Job drawing, mm, ordinate dimensions from the low corner. One solid piece. Coordinates: 2 decimals unless noted, no trailing zeros. Write each loop counter-clockwise with the first axis right and the second up, starting at its lowest first coordinate (ties: lowest second). Pieces come first, ordered by that corner, then holes. Notation, with made-up numbers: (53, 21) - (106, 21) arc R15 cw to (106, 45) - close; hole circle Ø8 at (24.5, -37). An arc over 180 degrees is marked (long way). Put each result on its own line as item: value. Start each with the question number.
1. Drill centre lines: L1, parallel to X at y = 1.25, z = 61; L2, parallel to Z at x = 72, y = 0.9; L3, parallel to Z at x = 52, y = 6.25. Where is each one in solid material? Low to high. Write a range as from..to.
2. Pull direction X, two halves, no side cores. Call the marked faces 1 and 2: released by +X, released by -X, zero draft, split by the parting line, or undercut.
3. Saw through at C-C, the plane x = 54. Write the cut outline in (y, z).
4. Saw through at A-A, the plane z = 61. Write the cut outline in (x, y).
5. Saw through at B-B, the plane x = 32. Write the cut outline in (y, z), plus the area to 3 significant figures.
6. Drop flat-ended pins along their axis: P1, Ø20, axis at x = 47.5, z = 56.5, coming from the +Y side; P2, Ø4, axis at x = 76, z = 45.5, coming from the -Y side; P3, Ø5, axis at x = 32, z = 61, coming from the +Y side; P4, Ø4, axis at x = 32, z = 77, coming from the +Y side. Give the stop position or say it passes through.
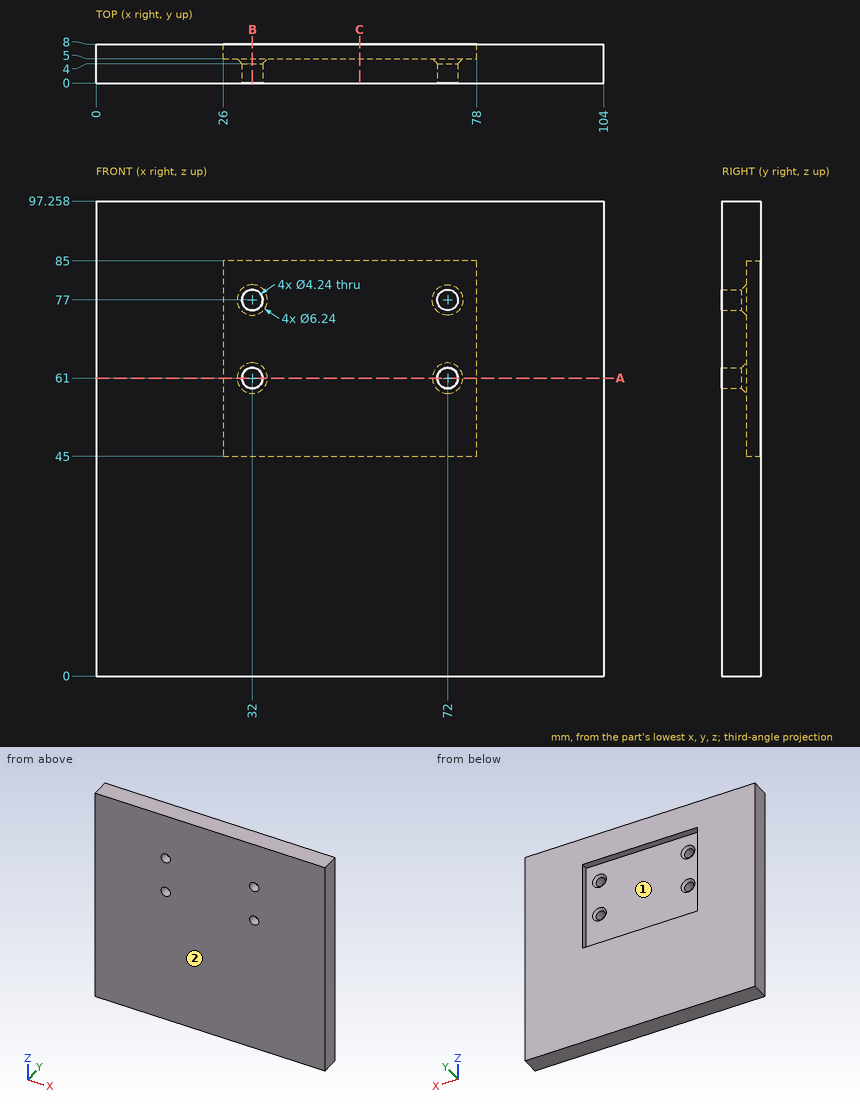
Final values:
1. L1: x = 0..29.88, 34.12..69.88, 74.12..104
1. L2: z = 0..58.88, 63.12..74.88, 79.12..97.26
1. L3: z = 0..45, 85..97.26
2. face 1: undercut
2. face 2: zero draft
3. outline: (0, 0) - (8, 0) - (8, 45) - (5, 45) - (5, 85) - (8, 85) - (8, 97.26) - (0, 97.26) - close
4. outline: (0, 0) - (29.88, 0) - (29.88, 4) - (28.88, 5) - (26, 5) - (26, 8) - (0, 8) - close; (34.12, 0) - (69.88, 0) - (69.88, 4) - (68.88, 5) - (35.12, 5) - (34.12, 4) - close; (74.12, 0) - (104, 0) - (104, 8) - (78, 8) - (78, 5) - (75.12, 5) - (74.12, 4) - close
5. outline: (0, 0) - (8, 0) - (8, 45) - (5, 45) - (5, 57.88) - (4, 58.88) - (0, 58.88) - close; (0, 63.12) - (4, 63.12) - (5, 64.12) - (5, 73.88) - (4, 74.88) - (0, 74.88) - close; (0, 79.12) - (4, 79.12) - (5, 80.12) - (5, 85) - (8, 85) - (8, 97.26) - (0, 97.26) - close
5. area: 614 mm²
6. P1: stops at y = 5
6. P2: stops at y = 0
6. P3: stops at y = 4.38
6. P4: passes through
